Geometry check sheet. Reference: the model listing, model coordinates, mm. Face numbers are marked on the shaded views. A direction names the side the tool comes from. Give positions to 0.01 mm unless a question says otherwise; leave off trailing zeros. Loops run counter-clockwise (first coordinate to the right, second up) from the corner with the lowest first, then second, coordinate; pieces in that order, holes last. Notation, with made-up numbers: (45.25, 19.5) - (58.25, 19.5) arc R25 cw to (58.25, 51.5) - close; hole circle Ø8 at (-38, 52.5). An arc over 180 degrees is marked (long way). Use a Markdown table: item, result. Add a question column.
1. Cross-section at C-C on x = 20. Enter the section's corners in (y, z).
2. Set-up check for the marked faces 1, 2 and 3: record each of +Z, -Z, +X, -X, +Y, -Y from which the full face is reachable in a straight line by a thin tool's end or side.
3. Material ranges on L1, parallel to Y at x = 81, z = 0; L2, parallel to X at y = -8.25, z = 0.5; L3, parallel to Y at x = 73, z = 8, recorded low to high.
4. Cross-section at B-B on y = 0. Enter the section's corners in (x, z), and give its area (3 significant figures).
5. Cross-section at D-D on y = -5. Enter the section's corners in (x, z) (3 decimals), and give its area (3 significant figures).
6. Cross-section at A-A on z = 0. Enter the section's corners in (x, y).
7. Depth check by flat-ended pin: P1, Ø4, axis at y = -7, z = 7, coming from the -X side; P2, Ø1.8, axis at x = 82, y = 1.5, coming from the +Z side; P3, Ø0.7, axis at x = 80.5, z = 7.5, coming from the -Y side; P4, Ø12, axis at x = 70.5, z = 3, coming from the -Y side. Enter the tip coordinate at first touch or a pass-through.
from build123d import *

# Parameters (mm, degrees)
CUT_EXTRUDE_2_DEPTH = 3


with BuildPart() as part:
    # 草图2 → 旋转1 (revolve)
    with BuildSketch(Plane(origin=(0, 0, 0), x_dir=(1, 0, 0), z_dir=(0, 1, 0))):
        Polygon((0, 0), (0, 8), (15, 8), (15, 9), (92, 9), (92, 10), (98, 10), (98, 9), (106, 9), (106, 0), align=None)
    revolve(axis=Axis((0, 0, 0), (1, 0, 0)))

    # 草图4 → 切除-拉伸2 (cut)
    with BuildSketch(Plane.XY.offset(9)):
        with BuildLine():
            Line((62, 3), (87, 3))
            ThreePointArc((87, 3), (90, 0), (87, -3))
            Line((87, -3), (62, -3))
            ThreePointArc((62, -3), (59, 0), (62, 3))
        make_face()
    extrude(amount=-CUT_EXTRUDE_2_DEPTH, mode=Mode.SUBTRACT)


solid = part.part
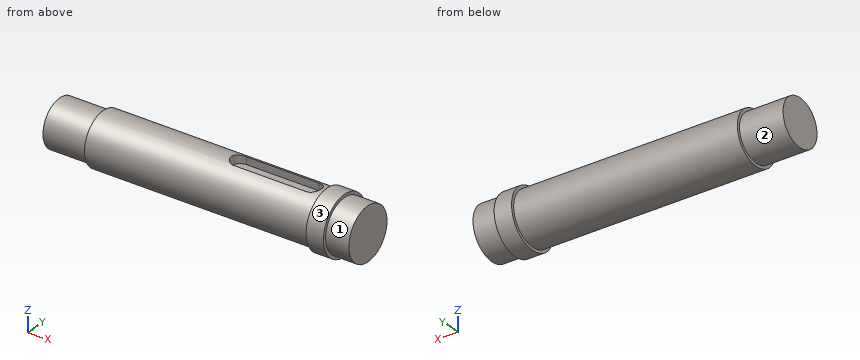
Values found:
| question | item | result |
|---|---|---|
| 1 | outline | circle Ø18 at (0, 0) |
| 2 | face 1 | +X |
| 2 | face 2 | -X |
| 2 | face 3 | +X, -X |
| 3 | L1 | y = -9 to 9 |
| 3 | L2 | x = 15 to 106 |
| 3 | L3 | y = -4.12 to -3, 3 to 4.12 |
| 4 | outline | (0, -8) - (15, -8) - (15, -9) - (92, -9) - (92, -10) - (98, -10) - (98, -9) - (106, -9) - (106, 9) - (98, 9) - (98, 10) - (92, 10) - (92, 9) - (90, 9) - (90, 6) - (59, 6) - (59, 9) - (15, 9) - (15, 8) - (0, 8) - close |
| 4 | area | 1,800 mm2 |
| 5 | outline | (0, -6.245) - (15, -6.245) - (15, -7.483) - (92, -7.483) - (92, -8.66) - (98, -8.66) - (98, -7.483) - (106, -7.483) - (106, 7.483) - (98, 7.483) - (98, 8.66) - (92, 8.66) - (92, 7.483) - (15, 7.483) - (15, 6.245) - (0, 6.245) - close |
| 5 | area | 1,560 mm2 |
| 6 | outline | (0, -8) - (15, -8) - (15, -9) - (92, -9) - (92, -10) - (98, -10) - (98, -9) - (106, -9) - (106, 9) - (98, 9) - (98, 10) - (92, 10) - (92, 9) - (15, 9) - (15, 8) - (0, 8) - close |
| 7 | P1 | stops at x = 0 |
| 7 | P2 | stops at z = 6 |
| 7 | P3 | stops at y = -5.47 |
| 7 | P4 | stops at y = -9 |
